```python
from build123d import *

# Parameters (mm, degrees)
ESTRUSIONE_ESTRUSIONE1_DEPTH = 30
SVUOTA4_DEPTH                = 30
SCHIZZO2_R                   = 45.510557865
SCHIZZO2_R_2                 = 3
ESTRUSIONE_ESTRUSIONE2_DEPTH = 2
FORO_PER_VITE_5_16_1_D       = 8.4328
FORO_PER_VITE_5_16_1_DEPTH   = 5


# Read off the part's stored shape, not the designer's step: Svuota4
with BuildPart() as part:
    # Schizzo1 → Estrusione-Estrusione1 (new body)
    with BuildSketch(Plane(origin=(0, 0, 0), x_dir=(0, 0, -1), z_dir=(1, 0, 0))):
        with BuildLine():
            Line((-45.401622395, 0), (-26.054049287, 0))
            Line((-26.054049287, 0), (-26.054049287, -37.181901939))
            ThreePointArc((-26.054049287, -37.181901939), (41.721933403, -17.904959905), (9, 44.500643996))
            Line((9, 44.500643996), (9, 14.325779192))
            Line((9, 14.325779192), (-9, 14.325779192))
            Line((-9, 14.325779192), (-9, 44.500643996))
            ThreePointArc((-9, 44.500643996), (-35.142011309, 28.74624075), (-45.401622395, 0))
        make_face()
    extrude(amount=ESTRUSIONE_ESTRUSIONE1_DEPTH)

    # Svuota4 outline → Svuota4 (cut)
    with BuildSketch(Plane.YZ):
        with BuildLine():
            Line((14.325779192, -14), (14.325779192, 14))
            Line((14.325779192, 14), (37.898431262, 14))
            ThreePointArc((37.898431262, 14), (25.104867632, 31.654963486), (5, 40.091035059))
            Line((5, 40.091035059), (5, 21.054049287))
            Line((5, 21.054049287), (-34.482141765, 21.054049287))
            ThreePointArc((-34.482141765, 21.054049287), (-17.610063922, -36.361748319), (37.898431262, -14))
            Line((37.898431262, -14), (14.325779192, -14))
        make_face()
    extrude(amount=SVUOTA4_DEPTH, mode=Mode.SUBTRACT)

    # Schizzo2 → Estrusione-Estrusione2 (add)
    with BuildSketch(Plane.ZY):
        Circle(SCHIZZO2_R)
        Circle(SCHIZZO2_R_2, mode=Mode.SUBTRACT)
    extrude(amount=ESTRUSIONE_ESTRUSIONE2_DEPTH)

    # Foro per Vite 5/16-1
    with Locations(Plane(origin=(15, -23.530287744, 26.054049287), x_dir=(0, 1, 0), z_dir=(0, 0, 1))):
        with Locations((0, 0)):
            Hole(FORO_PER_VITE_5_16_1_D / 2, depth=FORO_PER_VITE_5_16_1_DEPTH)


solid = part.part
```
For this review, take the finished solid that the model builds, in its own axes (mm). A direction names the side the tool comes from. Round coordinates to 2 decimals unless told otherwise and drop trailing zeros. Write each loop counter-clockwise with the first axis right and the second up, starting at its lowest first coordinate (ties: lowest second). Pieces come first, ordered by that corner, then holes. Notation, with made-up numbers: (76.25, -35.75) - (124.25, -35.75) arc R19 ccw to (124.25, -4.75) - close; hole circle Ø4 at (9, 46.5). An arc over 180 degrees is marked (long way). Answer as CSV lines item,"result". Start each with the question number.
(1) For pin 1 (5 mm diameter, centred on x = 15, y = -23.53, fed in from +Z); pin 2 (2.5 mm diameter, centred on x = 10, z = 10.5, fed in from -Y); pin 3 (1 mm diameter, centred on y = -7, z = -33.5, fed in from +X), all flat-tipped, find the tip position at first contact; note any pin that passes through.
(2) Mouldability with a two-part tool opening along Y and no side actions: class faces 1 (the flat face through (30, 16, -10)), 2 (the flat face through (15, 26, -14)), 3 (the cylindrical face through (14.79, -18.937, -41.264)) as +Y half, -Y half, draft (parallel to the pull), parting line (faces both ways), or undercut.
(3) Machinability: for faces 4 (the cylindrical face through (14.79, 29.082, 34.864)), 5 (the flat face through (15, 14.326, -12)), 6 (the flat face through (15, 0, 36)), 7 (the flat face through (15, 30, -9)), which of the approach directions +Z, -Z, +X, -X, +Y, -Y give a long, thin tool a straight path to every point of the face, cutting with its end or side? Answer none if there is none.
(4) Add section A-A, the plane x = 17. State the section outline as (y, z) points, plus the area to 3 significant figures.
(5) Add section C-C, the plane x = 27. State the section outline as (y, z) points.
(6) For line 1 (Z direction, x = 1, y = 36.5); line 2 (Y direction, x = -0.4, z = 0); line 3 (Z direction, x = 25, y = -29.5), list the stretches that pass through material, from the lowest coordinate up.
(7) Add section D-D, the plane y = -30.5. State the section outline as (x, z) points, plus the area to 3 significant figures.
(8) Add section B-B, the plane z = -1.5. State the section outline as (x, y) points, plus the area to 3 significant figures.
From the geometry:
1,pin 1,"stops at z = -30.9"
1,pin 2,"stops at y = -44.45"
1,pin 3,"stops at x = 0"
2,face 1,"draft"
2,face 2,"undercut"
2,face 3,"parting line"
3,face 4,"+Z, +X, +Y"
3,face 5,"+X"
3,face 6,"+Z, +X, -Y"
3,face 7,"+X, +Y"
4,outline,"(-37.18, 26.05) arc R45.4 ccw (long way) to (44.5, -9) - (14.33, -9) - (14.33, -14) - (37.9, -14) arc R40.4 cw (long way) to (-34.48, 21.05) - (-27.24, 21.05) - (-27.24, 26.05) - close; (-19.82, 21.05) - (5, 21.05) - (5, 40.09) arc R40.4 cw to (37.9, 14) - (14.33, 14) - (14.33, 9) - (44.5, 9) arc R45.4 ccw to (0, 45.4) - (0, 26.05) - (-19.82, 26.05) - close"
4,area,"1,530 mm²"
5,outline,"(-37.18, 26.05) arc R45.4 ccw (long way) to (44.5, -9) - (14.33, -9) - (14.33, -14) - (37.9, -14) arc R40.4 cw (long way) to (-34.48, 21.05) - (5, 21.05) - (5, 40.09) arc R40.4 cw to (37.9, 14) - (14.33, 14) - (14.33, 9) - (44.5, 9) arc R45.4 ccw to (0, 45.4) - (0, 26.05) - close"
6,line 1,"z = -27 to -17.32, -14 to -9, 9 to 14, 17.32 to 27"
6,line 2,"y = -45.51 to -3, 3 to 45.51"
6,line 3,"z = -34.51 to -27.61, 21.05 to 26.05"
7,outline,"(-2, -33.78) - (0, -33.78) - (0, -33.63) - (30, -33.63) - (30, -26.5) - (0, -26.5) - (0, 21.05) - (30, 21.05) - (30, 26.05) - (0, 26.05) - (0, 33.78) - (-2, 33.78) - close"
7,area,"499 mm²"
8,outline,"(-2, -45.49) - (0, -45.49) - (0, -45.38) - (30, -45.38) - (30, -40.37) - (0, -40.37) - (0, -2.6) - (-2, -2.6) - close; (-2, 2.6) - (0, 2.6) - (0, 45.49) - (-2, 45.49) - close"
8,area,"322 mm²"
